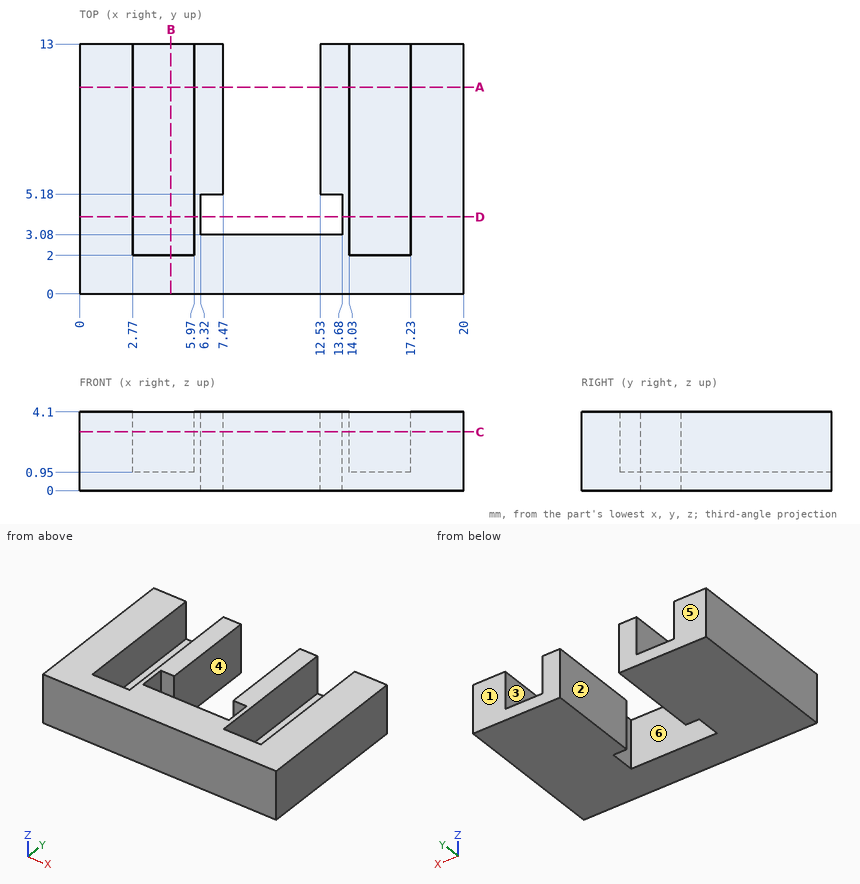
Study the drawing (mm; zero at the part's minimum x, y, z) and answer. A direction names the side the tool comes from. Give positions to 0.01 mm unless a question says otherwise; leave off trailing zeros. Loops run counter-clockwise (first coordinate to the right, second up) from the corner with the lowest first, then second, coordinate; pieces in that order, holes last. Notation, with made-up numbers: (38, 24.25) - (87, 24.25) arc R29 cw to (87, 50.25) - close; hole circle Ø9 at (53, 24.5). An arc over 180 degrees is marked (long way). Answer in a Markdown table with one row per item. Add a question column.
Q1. The part is cut by section D-D (y = 4). Determine the outline of the cut face in (x, z).
Q2. This flat-tipped pin is pushed along its axis until it touches: P1, Ø1, axis at x = 4.5, y = 10, coming from the +Z side. Where does it stop, or does it pass through?
Q3. A tool of negligible diameter and unlimited length cuts with its end or side. For the marked faces 1, 2 and 3, from which of +Z, -Z, +X, -X, +Y, -Y can it reach the whole face along a straight path? Write none if from no direction.
Q4. The part is cut by section B-B (x = 4.75). Determine the outline of the cut face in (y, z).
Q5. Consider line 1 along X through (y, z) = (10.25, 3.5); line 2 along X through (y, z) = (5, 2.5); line 3 along Y through (x, z) = (7, 0.2). Determine where each line is inside the solid, lowest interval first.
Q6. The part is cut by section A-A (y = 10.75). Determine the outline of the cut face in (x, z).
Q7. Determine the mould class of the marked faces 4, 5 and 6 for opening direction Y: released by +Y, released by -Y, zero draft, split by the parting line, or undercut.
Q8. The part is cut by section C-C (z = 3.05). Determine the outline of the cut face in (x, y).
Solution:
| question | item | result |
|---|---|---|
| 1 | outline | (0, 0) - (6.32, 0) - (6.32, 4.1) - (5.97, 4.1) - (5.97, 0.95) - (2.77, 0.95) - (2.77, 4.1) - (0, 4.1) - close; (13.68, 0) - (20, 0) - (20, 4.1) - (17.23, 4.1) - (17.23, 0.95) - (14.03, 0.95) - (14.03, 4.1) - (13.68, 4.1) - close |
| 2 | P1 | stops at z = 0.95 |
| 3 | face 1 | +Z, -Z, +X, -X, +Y |
| 3 | face 2 | +Z, -Z, +Y |
| 3 | face 3 | +Z, +Y |
| 4 | outline | (0, 0) - (13, 0) - (13, 0.95) - (2, 0.95) - (2, 4.1) - (0, 4.1) - close |
| 5 | line 1 | x = 0 to 2.77, 5.97 to 7.47, 12.53 to 14.03, 17.23 to 20 |
| 5 | line 2 | x = 0 to 2.77, 5.97 to 6.32, 13.68 to 14.03, 17.23 to 20 |
| 5 | line 3 | y = 0 to 3.08, 5.18 to 13 |
| 6 | outline | (0, 0) - (7.47, 0) - (7.47, 4.1) - (5.97, 4.1) - (5.97, 0.95) - (2.77, 0.95) - (2.77, 4.1) - (0, 4.1) - close; (12.53, 0) - (20, 0) - (20, 4.1) - (17.23, 4.1) - (17.23, 0.95) - (14.03, 0.95) - (14.03, 4.1) - (12.53, 4.1) - close |
| 7 | face 4 | zero draft |
| 7 | face 5 | released by +Y |
| 7 | face 6 | undercut |
| 8 | outline | (0, 0) - (20, 0) - (20, 13) - (17.23, 13) - (17.23, 2) - (14.03, 2) - (14.03, 13) - (12.53, 13) - (12.53, 5.18) - (13.68, 5.18) - (13.68, 3.08) - (6.32, 3.08) - (6.32, 5.18) - (7.47, 5.18) - (7.47, 13) - (5.97, 13) - (5.97, 2) - (2.77, 2) - (2.77, 13) - (0, 13) - close |
